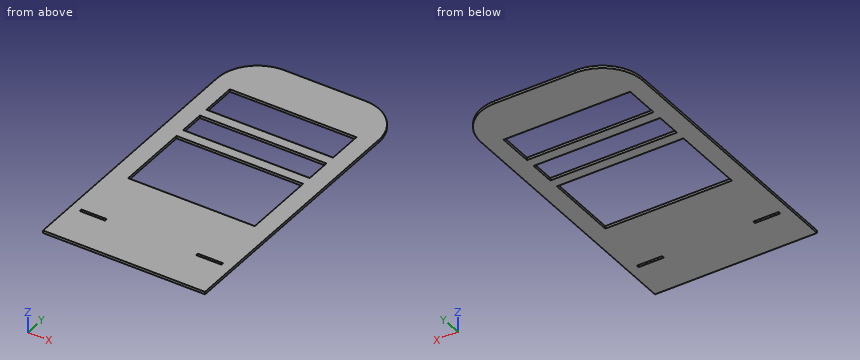
```python
from build123d import *

# Parameters (mm, degrees)
F0_W     = 127
F0_H     = 12.7
F0_W_2   = 635
F0_H_2   = 126.9999911487
F0_H_3   = 177.8000088513
F1_DEPTH = 12.7


# Not quite as in the source:
# - a feature names something its author has since deleted; it is built from what else it names


with BuildPart() as f1:
    # F0 (on Top) → F1 (new body)
    with BuildSketch(Plane.XY):
        with BuildLine():
            ThreePointArc((-444.8386187891, 967.019580251), (-588.5227167262, 907.5036781881), (-648.0386187891, 763.819580251))
            Line((-648.0386187891, 763.819580251), (-648.0386187891, -556.980419749))
            Line((-648.0386187891, -556.980419749), (-648.0386187891, -563.330419749))
            Line((-648.0386187891, -563.330419749), (164.7613812109, -563.330419749))
            Line((164.7613812109, -563.330419749), (164.7613812109, -556.980419749))
            Line((164.7613812109, -556.980419749), (164.7613812109, 763.819580251))
            ThreePointArc((164.7613812109, 763.819580251), (105.245479148, 907.5036781881), (-38.4386187891, 967.019580251))
            Line((-38.4386187891, 967.019580251), (-444.8386187891, 967.019580251))
        make_face()
        with Locations((-533.7386187891, -353.780419749)):
            Rectangle(F0_W, F0_H, mode=Mode.SUBTRACT)
        with Locations((50.4613812109, -353.780419749)):
            Rectangle(F0_W, F0_H, mode=Mode.SUBTRACT)
        Polygon((75.8613812109, -48.980419749), (-559.1386187891, -48.980419749), (-559.1386187891, 90.719580251), (-559.1386187891, 141.519580251), (-559.1386187891, 319.319580251), (75.8613812109, 319.319580251), (75.8613812109, 141.519580251), (75.8613812109, 90.719580251), align=None, mode=Mode.SUBTRACT)
        with Locations((-241.6386187891, 433.6195758253)):
            Rectangle(F0_W_2, F0_H_2, mode=Mode.SUBTRACT)
        with Locations((-241.6386187891, 636.8195758253)):
            Rectangle(F0_W_2, F0_H_3, mode=Mode.SUBTRACT)
    extrude(amount=F1_DEPTH)


solid = f1.part
```
Here's how the part is built. I have some questions about the finished solid (model axes, mm). Give positions to 0.01 mm unless a question says otherwise; leave off trailing zeros. Order: outer loops, then holes, each group sorted by start corner. A loop starts at its lowest first (then second) coordinate and runs counter-clockwise, first axis right, second up. Notation, with made-up numbers: (53.25, 33) - (84.25, 33) arc R12 ccw to (84.25, 49) - close; hole circle Ø4 at (11, -14). An arc over 180 degrees is marked (long way). Answer as a JSON object with one key per item and string values. Group by question number.
Item 1: If we section it at D-D on x = -581.5: Please give me the cut outline in (y, z), and give its area (3 significant figures).
Item 2: If we section it at A-A on x = -181.5: Please give me the cut outline in (y, z), and give its area (3 significant figures).
Item 3: If we section it at B-B on y = 84: Please give me the cut outline in (x, z).
Item 4: If we section it at C-C on z = 5.5: Please give me the cut outline in (x, y), and give its area (4 significant figures).
Item 5: For P1, Ø8, axis at x = -505.5, y = 812, coming from the -Z side; P2, Ø6.5, axis at x = 22, z = 6, coming from the +Y side; P3, Ø1.5, axis at x = 30.5, z = 5.5, coming from the +Y side; P4, Ø4, axis at x = -559.5, z = 5.5, coming from the +Y side, each with a flat end and sliding along its axis, tell me the tip position at first contact or that it passes through.
Item 6: Please list where these lines run through material, in increasing order: probe 1 along Y at (x, z) = (-37.5, 6); probe 2 along X at (y, z) = (638.5, 2); probe 3 along Y at (x, z) = (-534, 1.5).
Result set:
{
 "1": {"outline": "(-563.33, 0) - (-360.13, 0) - (-360.13, 12.7) - (-563.33, 12.7) - close; (-347.43, 0) - (914.2, 0) - (914.2, 12.7) - (-347.43, 12.7) - close", "area": "18,600 mm²"},
 "2": {"outline": "(-563.33, 0) - (-48.98, 0) - (-48.98, 12.7) - (-563.33, 12.7) - close; (319.32, 0) - (370.12, 0) - (370.12, 12.7) - (319.32, 12.7) - close; (497.12, 0) - (547.92, 0) - (547.92, 12.7) - (497.12, 12.7) - close; (725.72, 0) - (967.02, 0) - (967.02, 12.7) - (725.72, 12.7) - close", "area": "10,900 mm²"},
 "3": {"outline": "(-648.04, 0) - (-559.14, 0) - (-559.14, 12.7) - (-648.04, 12.7) - close; (75.86, 0) - (164.76, 0) - (164.76, 12.7) - (75.86, 12.7) - close"},
 "4": {"outline": "(-648.04, -563.33) - (164.76, -563.33) - (164.76, 763.82) arc R203.2 ccw to (-38.44, 967.02) - (-444.84, 967.02) arc R203.2 ccw to (-648.04, 763.82) - close; hole (-597.24, -360.13) - (-470.24, -360.13) - (-470.24, -347.43) - (-597.24, -347.43) - close; hole (-559.14, -48.98) - (75.86, -48.98) - (75.86, 319.32) - (-559.14, 319.32) - close; hole (-559.14, 370.12) - (75.86, 370.12) - (75.86, 497.12) - (-559.14, 497.12) - close; hole (-559.14, 547.92) - (75.86, 547.92) - (75.86, 725.72) - (-559.14, 725.72) - close; hole (-13.04, -360.13) - (113.96, -360.13) - (113.96, -347.43) - (-13.04, -347.43) - close", "area": "795,500 mm²"},
 "5": {"P1": "z = 0", "P2": "y = 958.81", "P3": "y = 955.24", "P4": "y = 932.93"},
 "6": {"probe 1": "-563.33 to -48.98, 319.32 to 370.12, 497.12 to 547.92, 725.72 to 967.02", "probe 2": "-648.04 to -559.14, 75.86 to 164.76", "probe 3": "-563.33 to -360.13, -347.43 to -48.98, 319.32 to 370.12, 497.12 to 547.92, 725.72 to 946.41"}
}
